```python
from build123d import *

# Parameters (mm, degrees)
F0_W     = 127
F0_H     = 50.8
F1_DEPTH = 85.09
F3_R     = 13.5622431152
F4_DEPTH = 73.914


with BuildPart() as f1:
    # F0 (on Front) → F1 (new body)
    with BuildSketch(Plane.XZ):
        with Locations((-36.1398326457, 12.9770052895)):
            Rectangle(F0_W, F0_H)
    extrude(amount=F1_DEPTH)

    # F3 (on face) → F4 (cut)
    with BuildSketch(Plane.XY.offset(38.3770052895)):
        with Locations((-55.075917393, -34.1837741435)):
            Circle(F3_R)
    extrude(amount=-F4_DEPTH, mode=Mode.SUBTRACT)


solid = f1.part
```
Work out the finished part from the listing and answer in its coordinate system (mm). Round coordinates to 2 decimals unless told otherwise and drop trailing zeros. Loops run counter-clockwise (first coordinate to the right, second up) from the corner with the lowest first, then second, coordinate; pieces in that order, holes last.
(1) The part is cut by section B-B, the plane x = -47. Give the vertices of the cut face in (y, z), and give its area (3 significant figures).
Computed values:
outline: (-85.09, -12.42) - (-45.08, -12.42) - (-45.08, 38.38) - (-85.09, 38.38) - close; (-23.29, -12.42) - (0, -12.42) - (0, 38.38) - (-23.29, 38.38) - close
area: 3,220 mm2
(2) The mould has two halves that part along X. Classify faces 1 (the flat face through (-99.64, -42, 13)), 2 (the flat face through (-37, 0, 13)), 3 (the flat face through (27.36, -42, 13)), 4 (the cylindrical face through (-65.838, -42.436, 13.333)): pulls with the +X half, pulls with the -X half, needs draft (parallel to the pull), parting line crosses it, or undercut.
Computed values:
face 1: pulls with the -X half
face 2: needs draft
face 3: pulls with the +X half
face 4: undercut
(3) The part is cut by section C-C, the plane z = 5. Give the vertices of the cut face in (x, y).
Computed values:
outline: (-99.64, -85.09) - (27.36, -85.09) - (27.36, 0) - (-99.64, 0) - close; hole circle Ø27.12 at (-55.08, -34.18)
(4) Find the intervals of material crossed by L1, parallel to X at y = -34, z = 33; L2, parallel to X at y = -22, z = -3; L3, parallel to Y at x = -62, z = 23, in increasing order.
Computed values:
L1: x = -99.64 to -68.64, -41.51 to 27.36
L2: x = -99.64 to -61.03, -49.12 to 27.36
L3: y = -85.09 to -45.85, -22.52 to 0
(5) The part is cut by section A-A, the plane y = -26. Give the vertices of the cut face in (x, z), and give its area (3 significant figures).
Computed values:
outline: (-99.64, -12.42) - (-65.89, -12.42) - (-65.89, 38.38) - (-99.64, 38.38) - close; (-44.26, -12.42) - (27.36, -12.42) - (27.36, 38.38) - (-44.26, 38.38) - close
area: 5,350 mm2
